For this review, use the dimensioned drawing (mm, ordinates from the lowest corner) and the shaded views. Give positions to 0.01 mm unless a question says otherwise; leave off trailing zeros. Loops run counter-clockwise (first coordinate to the right, second up) from the corner with the lowest first, then second, coordinate; pieces in that order, holes last. Notation, with made-up numbers: (-24, 48) - (-8, 48) arc R26 ccw to (-8, 69) - close; hole circle Ø2 at (32.5, 8.25). An arc over 180 degrees is marked (long way). Put each result on its own line as item: value.
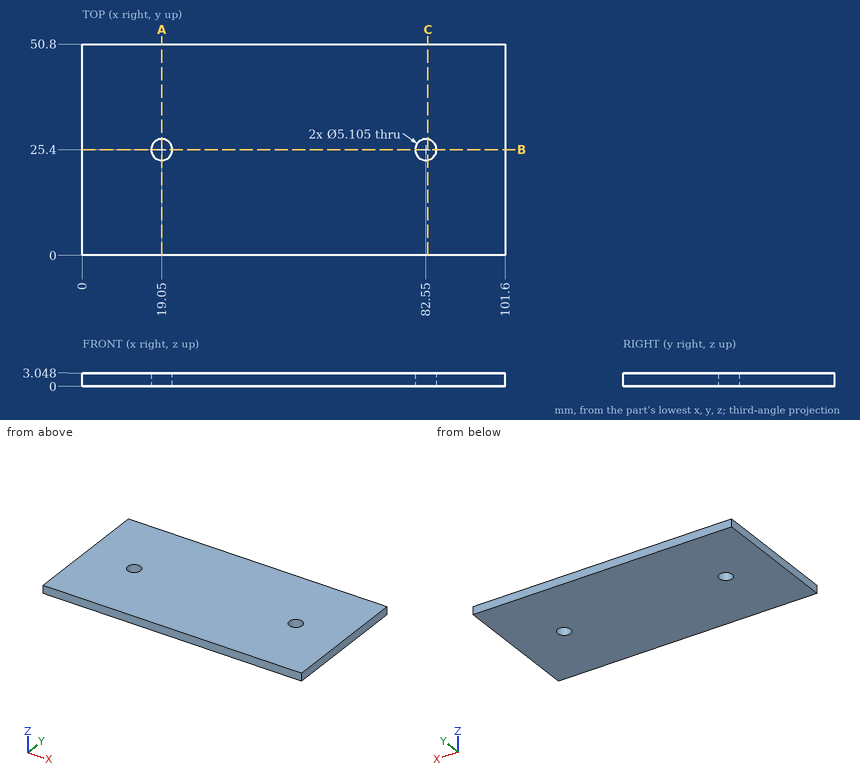
1) Wall thickness on line 1 (Y direction, x = 82.55, z = 0.7); line 2 (Y direction, x = 18, z = 0.3): over which ranges is each line inside the solid? List them lowest first.
Geometry check:
line 1: y = 0 to 22.85, 27.95 to 50.8
line 2: y = 0 to 23.07, 27.73 to 50.8
2) Take a section at B-B on y = 25.4. State the section outline as (x, z) points.
Geometry check:
outline: (0, 0) - (16.5, 0) - (16.5, 3.05) - (0, 3.05) - close; (21.6, 0) - (80, 0) - (80, 3.05) - (21.6, 3.05) - close; (85.1, 0) - (101.6, 0) - (101.6, 3.05) - (85.1, 3.05) - close
3) Take a section at A-A on x = 19.05. State the section outline as (y, z) points, and give its area (3 significant figures).
Geometry check:
outline: (0, 0) - (22.85, 0) - (22.85, 3.05) - (0, 3.05) - close; (27.95, 0) - (50.8, 0) - (50.8, 3.05) - (27.95, 3.05) - close
area: 139 mm²
4) Take a section at C-C on x = 83. State the section outline as (y, z) points.
Geometry check:
outline: (0, 0) - (22.89, 0) - (22.89, 3.05) - (0, 3.05) - close; (27.91, 0) - (50.8, 0) - (50.8, 3.05) - (27.91, 3.05) - close
5) Insertion check: pin 1 Ø4 at (x, y) = (19.05, 25.4) entering from +Z. The pin has a flat end and moves straight along its axis. Give the tip position at first contact, or say it passes through.
Geometry check:
pin 1: passes through
